Design review of the part built by this model. Coordinates are the model's own, in mm. Give positions to 0.01 mm unless a question says otherwise; leave off trailing zeros. Order: outer loops, then holes, each group sorted by start corner. A loop starts at its lowest first (then second) coordinate and runs counter-clockwise, first axis right, second up. Notation, with made-up numbers: M 51,15 L 66,15 A11 cw 66,36 Z; hole C -14.75,19 d6. An arc over 180 degrees is marked long. Answer as a JSON object with one key per item and string values.
from build123d import *

# Parameters (mm, degrees)
F1_DEPTH = 12.7
F2_R     = 4.0005
F2_R_2   = 4
F3_DEPTH = 12.7


with BuildPart() as f1:
    # F0 (on Front) → F1 (new body)
    with BuildSketch(Plane.XZ):
        with BuildLine():
            Line((-13.8799677983, 7.9941251807), (-13.5483602062, 0))
            Line((-13.5483602062, 0), (-21.5493602062, 0))
            ThreePointArc((-21.5493602062, 0), (-19.2059215625, -5.6575613563), (-13.5483602062, -8.001))
            ThreePointArc((-13.5483602062, -8.001), (-7.8907988499, -5.6575613563), (-5.5473602062, 0))
            ThreePointArc((-5.5473602062, 0), (-5.5490811437, 0.1659381806), (-5.5542432158, 0.3318049778))
            ThreePointArc((-5.5542432158, 0.3318049778), (-8.13021474, 5.8872489932), (-13.8799677983, 7.9941251807))
        make_face()
        with BuildLine():
            Line((-14.8953476758, 32.4720745373), (-13.8799677983, 7.9941251807))
            ThreePointArc((-13.8799677983, 7.9941251807), (-8.13021474, 5.8872489932), (-5.5542432158, 0.3318049778))
            Line((-5.5542432158, 0.3318049778), (-7.2337959714, 40.7969640847))
            ThreePointArc((-7.2337959714, 40.7969640847), (-7.2286345445, 40.6311180182), (-7.2269138221, 40.4652005773))
            ThreePointArc((-7.2269138221, 40.4652005773), (-9.4540233342, 34.9268131392), (-14.8953476758, 32.4720745373))
        make_face()
        with BuildLine():
            Line((-15.2269138221, 40.4652005773), (-14.8953476758, 32.4720745373))
            ThreePointArc((-14.8953476758, 32.4720745373), (-9.4540233342, 34.9268131392), (-7.2269138221, 40.4652005773))
            ThreePointArc((-7.2269138221, 40.4652005773), (-7.2286345445, 40.6311180182), (-7.2337959714, 40.7969640847))
            ThreePointArc((-7.2337959714, 40.7969640847), (-12.4160884571, 47.9551445535), (-21.0282775518, 45.9737556397))
            ThreePointArc((-21.0282775518, 45.9737556397), (-23.2242322391, 40.2580819225), (-20.7353649166, 34.6637381289))
            Line((-20.7353649166, 34.6637381289), (-15.2269138221, 40.4652005773))
        make_face()
        with BuildLine():
            Line((-48.1392205553, 5.8021876312), (-20.7353649166, 34.6637381289))
            ThreePointArc((-20.7353649166, 34.6637381289), (-23.2242322391, 40.2580819225), (-21.0282775518, 45.9737556397))
            Line((-21.0282775518, 45.9737556397), (-59.4504491063, 5.5092436318))
            ThreePointArc((-59.4504491063, 5.5092436318), (-53.8555047508, 7.9983180818), (-48.1392205553, 5.8021876312))
        make_face()
        with BuildLine():
            ThreePointArc((-53.6483602062, -8.001), (-47.9907988499, -5.6575613563), (-45.6473602062, 0))
            Line((-45.6473602062, 0), (-53.6483602062, 0))
            Line((-53.6483602062, 0), (-48.1392205553, 5.8021876312))
            ThreePointArc((-48.1392205553, 5.8021876312), (-53.8555047508, 7.9983180818), (-59.4504491063, 5.5092436318))
            ThreePointArc((-59.4504491063, 5.5092436318), (-61.0000763085, -3.1572569346), (-53.6483602062, -8.001))
        make_face()
        with BuildLine():
            ThreePointArc((-13.5483602062, -8.001), (-19.2059215625, -5.6575613563), (-21.5493602062, 0))
            Line((-21.5493602062, 0), (-45.6473602062, 0))
            ThreePointArc((-45.6473602062, 0), (-47.9907988499, -5.6575613563), (-53.6483602062, -8.001))
            Line((-53.6483602062, -8.001), (-13.5483602062, -8.001))
        make_face()
        with BuildLine():
            ThreePointArc((-21.5493602062, 0), (-19.3219723054, 5.5390797365), (-13.8799677983, 7.9941251807))
            Line((-13.8799677983, 7.9941251807), (-14.8953476758, 32.4720745373))
            ThreePointArc((-14.8953476758, 32.4720745373), (-18.0377645415, 32.975266116), (-20.7353649166, 34.6637381289))
            Line((-20.7353649166, 34.6637381289), (-48.1392205553, 5.8021876312))
            ThreePointArc((-48.1392205553, 5.8021876312), (-46.296672395, 3.15732281), (-45.6473602062, 0))
            Line((-45.6473602062, 0), (-21.5493602062, 0))
        make_face()
        with BuildLine():
            ThreePointArc((-20.7353649166, 34.6637381289), (-18.0377645415, 32.975266116), (-14.8953476758, 32.4720745373))
            Line((-14.8953476758, 32.4720745373), (-15.2269138221, 40.4652005773))
            Line((-15.2269138221, 40.4652005773), (-20.7353649166, 34.6637381289))
        make_face()
        with BuildLine():
            Line((-21.5493602062, 0), (-13.5483602062, 0))
            Line((-13.5483602062, 0), (-13.8799677983, 7.9941251807))
            ThreePointArc((-13.8799677983, 7.9941251807), (-19.3219723054, 5.5390797365), (-21.5493602062, 0))
        make_face()
        with BuildLine():
            Line((-53.6483602062, 0), (-45.6473602062, 0))
            ThreePointArc((-45.6473602062, 0), (-46.296672395, 3.15732281), (-48.1392205553, 5.8021876312))
            Line((-48.1392205553, 5.8021876312), (-53.6483602062, 0))
        make_face()
    extrude(amount=F1_DEPTH)

    # F2 (on face) → F3 (cut, through all)
    with BuildSketch(Plane.XZ.offset(12.7)):
        with Locations((-15.2269138221, 40.4652005773)):
            Circle(F2_R)
        with Locations((-13.5483602062, 0)):
            Circle(F2_R)
        with Locations((-53.6483602062, 0)):
            Circle(F2_R_2)
    extrude(amount=-F3_DEPTH, mode=Mode.SUBTRACT)


solid = f1.part
(1) We need section B-B (y = -5). Write out the cut boundary in (x, z).
Checked values:
{"outline": "M -59.45,5.51 A8 ccw -53.65,-8 L -13.55,-8 A8 ccw -5.55,0.33 L -7.23,40.8 A8 ccw -21.03,45.97 Z; hole C -53.65,0 d8; hole C -15.23,40.47 d8; hole C -13.55,0 d8"}
(2) Insertion check: pin 1 (4 mm diameter, centred on y = -6.5, z = 40.5, fed in from -X); pin 2 (1 mm diameter, centred on y = -9, z = 11.5, fed in from +X); pin 3 (1.5 mm diameter, centred on x = -29, y = -5, fed in from +Z). Each pin has a flat end and moves straight along its axis. Give the tip position at first contact, or say it passes through.
Checked values:
{"pin 1": "stops at x = -28.12", "pin 2": "stops at x = -6", "pin 3": "stops at z = 38.37"}
(3) We need section C-C (z = 24). Write out the cut boundary in (x, y), plus the area to 3 significant figures.
Checked values:
{"outline": "M -41.89,-12.7 L -6.54,-12.7 L -6.54,0 L -41.89,0 Z", "area": "449 mm^2"}
(4) We need section A-A (x = -16). Write out the cut boundary in (y, z).
Checked values:
{"outline": "M -12.7,-8 L 0,-8 L 0,-3.16 L -12.7,-3.16 Z; M -12.7,3.16 L 0,3.16 L 0,36.54 L -12.7,36.54 Z; M -12.7,44.39 L 0,44.39 L 0,48.43 L -12.7,48.43 Z"}
(5) We need section D-D (x = -31.5). Write out the cut boundary in (y, z).
Checked values:
{"outline": "M -12.7,-8 L 0,-8 L 0,34.95 L -12.7,34.95 Z"}
(6) Draft analysis for pull direction X (two halves, no side actions). For faces 1 (the cylindrical face through (-12.294, -6.261, 47.908)), 2 (the cylindrical face through (-13.381, -6.439, 36.916)), 3 (the flat face through (-6.382, -6.261, 20.281)), state which applies: +X half, -X half, draft (parallel to the pull), parting line (faces both ways), or undercut.
Checked values:
{"face 1": "parting line", "face 2": "undercut", "face 3": "+X half"}
(7) To check wall thickness, follow L1, parallel to X at y = -8, z = 1; L2, parallel to Z at x = -15, y = -11.5; L3, parallel to Z at x = -57, y = -3.5. State the ranges of each line that lie inside material, in increasing order. Write a range as from..to.
Checked values:
{"L1": "x = -61.59..-57.52, -49.78..-17.42, -9.67..-5.58", "L2": "z = -8..-3.73, 3.73..36.47, 44.46..48.46", "L3": "z = -7.27..-2.18, 2.18..8.09"}
